Part model, mm, in its own coordinate system. A direction names the side the tool comes from. Give positions to 0.01 mm unless a question says otherwise; leave off trailing zeros. Write each loop counter-clockwise with the first axis right and the second up, starting at its lowest first coordinate (ties: lowest second). Pieces come first, ordered by that corner, then holes. Notation, with made-up numbers: (-40, 44.25) - (9, 44.25) arc R34 ccw to (9, 76.25) - close; hole circle Ø2 at (9.5, 87.25). An arc over 180 degrees is marked (long way). Answer in a Markdown table with one row per item. Add a question column.
1. Drop flat-ended pins along their axis: pin 1 Ø5 at (x, y) = (-2.5, 12.5) entering from +Z; pin 2 Ø2.5 at (x, z) = (0.5, -1.5) entering from +Y; pin 3 Ø2.5 at (x, y) = (-1.5, 22.5) entering from +Z. Give the stop position or say it passes through.
2. Band-saw the part on B-B on x = -16. Write the cut outline in (y, z).
3. Band-saw the part on D-D on x = 11. Write the cut outline in (y, z).
4. Which spindle directions (+Z, -Z, +X, -X, +Y, -Y) get a long thin tool onto all of the face, cutting with end or side? Do faces 1 (the flat face through (2.095, 18.302, -20.986)), 2 (the flat face through (2.095, 4.014, 0.698)), 3 (the flat face through (-0.3, 5, 2.2)). Say none if no direction does.
5. Pull direction X, two halves, no side cores. Call faces 4 (the flat face through (-2.095, 25.698, -20.986)), 5 (the flat face through (0, 0, 0)), 6 (the flat face through (-21, 6, 19)): released by +X, released by -X, zero draft, split by the parting line, or undercut.
6. Band-saw the part on C-C on y = 51. Write the cut outline in (x, z).
7. Band-saw the part on A-A on y = 4. Write the cut outline in (x, z), plus the area to 3 significant figures.
8. Probe line 1 along X through (y, z) = (1.55, -3); line 2 along Y through (x, z) = (0, -24.1); line 3 along X through (y, z) = (37.5, -19.5). List the from-to ranges inside material, lowest first.
```python
from build123d import *

# Parameters (mm, degrees)
SKETCH1_W               = 50
SKETCH1_H               = 50
BOSS_EXTRUDE1_DEPTH     = 5
SKETCH2_W               = 50
SKETCH2_H               = 5
BOSS_EXTRUDE2_DEPTH     = 50
SKETCH3_R               = 2.6
CUT_EXTRUDE1_DEPTH      = 50
SKETCH4_R               = 2.6
CUT_EXTRUDE2_DEPTH      = 50
CHAMFER1_SIZE           = 10
CUT_EXTRUDE3_DEPTH      = 2
CUT_EXTRUDE4_DEPTH      = 2
BOSS_EXTRUDE3_DEPTH     = 5
BOSS_EXTRUDE4_START     = -50
BOSS_EXTRUDE4_DEPTH     = 5
CUT_EXTRUDE5_DEPTH      = 66.383484153
CUT_EXTRUDE5_DEPTH_BACK = 66.383484153
CUT_EXTRUDE6_DEPTH      = 79.421935707
CUT_EXTRUDE6_DEPTH_BACK = 79.421935707
FILLET1_R               = 4


with BuildPart() as part:
    # Sketch1 → Boss-Extrude1 (new body)
    with BuildSketch(Plane(origin=(0, 0, 0), x_dir=(1, 0, 0), z_dir=(0, 1, 0))):
        Rectangle(SKETCH1_W, SKETCH1_H)
    extrude(amount=BOSS_EXTRUDE1_DEPTH)

    # Sketch2 → Boss-Extrude2 (add)
    with BuildSketch(Plane(origin=(0, 5, 0), x_dir=(1, 0, 0), z_dir=(0, 1, 0))):
        with Locations((0, 22.5)):
            Rectangle(SKETCH2_W, SKETCH2_H)
    extrude(amount=BOSS_EXTRUDE2_DEPTH)

    # Sketch3 → Cut-Extrude1 (cut)
    with BuildSketch(Plane.XY.offset(-20)):
        with Locations((0, 22)):
            Circle(SKETCH3_R)
    extrude(amount=-CUT_EXTRUDE1_DEPTH, mode=Mode.SUBTRACT)

    # Sketch4 → Cut-Extrude2 (cut)
    with BuildSketch(Plane(origin=(0, 5, 0), x_dir=(1, 0, 0), z_dir=(0, 1, 0))):
        with Locations(Location((0, 3, 0), (0, 0, 270))):
            Circle(SKETCH4_R)
    extrude(amount=-CUT_EXTRUDE2_DEPTH, mode=Mode.SUBTRACT)

    # Chamfer1
    chamfer1_edges = [part.edges().sort_by_distance(p)[0] for p in [
        (25, 55, -22.5),
        (-25, 55, -22.5),
        (25, 2.5, 25),
        (-25, 2.5, 25),
    ]]
    chamfer(chamfer1_edges, length=CHAMFER1_SIZE)

    # Sketch5 → Cut-Extrude3 (cut)
    with BuildSketch(Plane.XY.offset(-20)):
        Polygon((0, 26.907477288), (-4.25, 24.453738644), (-4.25, 19.546261356), (0, 17.092522712), (4.25, 19.546261356), (4.25, 24.453738644), align=None)
    extrude(amount=-CUT_EXTRUDE3_DEPTH, mode=Mode.SUBTRACT)

    # Sketch6 → Cut-Extrude4 (cut)
    with BuildSketch(Plane(origin=(0, 5, 0), x_dir=(1, 0, 0), z_dir=(0, 1, 0))):
        Polygon((0, 7.907477288), (-4.25, 5.453738644), (-4.25, 0.546261356), (0, -1.907477288), (4.25, 0.546261356), (4.25, 5.453738644), align=None)
    extrude(amount=-CUT_EXTRUDE4_DEPTH, mode=Mode.SUBTRACT)

    # Sketch7 → Boss-Extrude3 (add)
    with BuildSketch(Plane.ZY.offset(25)):
        Polygon((-20, 55), (25, 5), (-20, 5), align=None)
    extrude(amount=-BOSS_EXTRUDE3_DEPTH)

    # Sketch7<2> → Boss-Extrude4 (add)
    with BuildSketch(Plane.ZY.offset(25).offset(BOSS_EXTRUDE4_START)):
        Polygon((-20, 55), (25, 5), (-20, 5), align=None)
    extrude(amount=BOSS_EXTRUDE4_DEPTH)

    # Sketch8 → Cut-Extrude5 (cut, two sides: drawn at the far end of the back side and taken through both)
    with BuildSketch(Plane.XZ.offset(-CUT_EXTRUDE5_DEPTH_BACK)):
        Polygon((-25, 15), (-15, 25), (15, 25), (25, 15), (34.688631102, 13.868509335), (41.480658752, 39.43849578), (-8.141096193, 43.673524785), (-46.895606899, 41.556010282), (-45.565833038, 17.218639636), (-29.396147425, 9.154043084), align=None)
    extrude(amount=CUT_EXTRUDE5_DEPTH + CUT_EXTRUDE5_DEPTH_BACK, mode=Mode.SUBTRACT)

    # Sketch9 → Cut-Extrude6 (cut, two sides: drawn at the far end of the back side and taken through both)
    with BuildSketch(Plane(origin=(0, 0, -25), x_dir=(-1, 0, 0), z_dir=(0, 0, -1)).offset(-CUT_EXTRUDE6_DEPTH_BACK)):
        Polygon((-25, 45), (-15, 55), (15, 55), (25, 45), (34.215912108, 41.57366901), (36.332651021, 61.374461749), (-31.078246872, 63.763955814), (-33.631649738, 52.638414759), (-28.038481557, 40.053786352), align=None)
    extrude(amount=CUT_EXTRUDE6_DEPTH + CUT_EXTRUDE6_DEPTH_BACK, mode=Mode.SUBTRACT)

    # Fillet1
    fillet1_edges = [part.edges().sort_by_distance(p)[0] for p in [
        (20, 30.277777778, 2.25),
        (-20, 30.277777778, 2.25),
    ]]
    fillet(fillet1_edges, radius=FILLET1_R)


solid = part.part
```
Values:
| question | item | result |
|---|---|---|
| 1 | pin 1 | stops at z = -20 |
| 1 | pin 2 | stops at y = 3 |
| 1 | pin 3 | stops at z = -22 |
| 2 | outline | (0, -25) - (54, -25) - (54, -20) - (5, -20) - (5, 24) - (0, 24) - close |
| 3 | outline | (0, -25) - (55, -25) - (55, -20) - (5, -20) - (5, 25) - (0, 25) - close |
| 4 | face 1 | +Z |
| 4 | face 2 | +Y |
| 4 | face 3 | +Z, +Y |
| 5 | face 4 | undercut |
| 5 | face 5 | zero draft |
| 5 | face 6 | released by -X |
| 6 | outline | (-19, -25) - (19, -25) - (19, -20) - (-19, -20) - close |
| 7 | outline | (-25, -25) - (25, -25) - (25, 15) - (15, 25) - (-15, 25) - (-25, 15) - close; hole (-4.25, -5.45) - (0, -7.91) - (4.25, -5.45) - (4.25, -0.55) - (0, 1.91) - (-4.25, -0.55) - close |
| 7 | area | 2,340 mm² |
| 8 | line 1 | x = -25 to -2.6, 2.6 to 25 |
| 8 | line 2 | y = 0 to 19.4, 24.6 to 55 |
| 8 | line 3 | x = -25 to -20, 20 to 25 |
